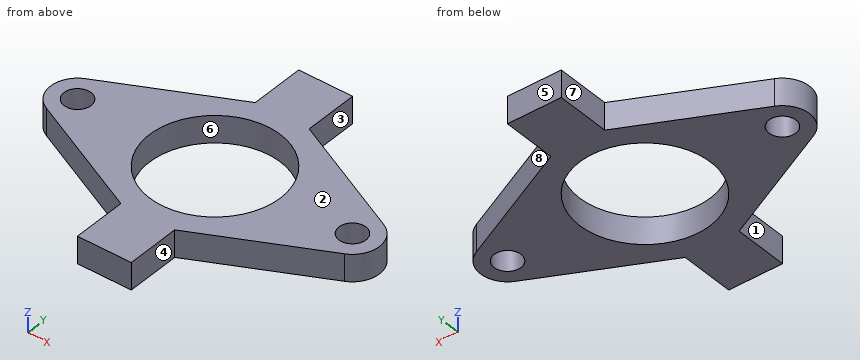
from build123d import *

# Parameters (mm, degrees)
SKETCH1_R           = 24.25
SKETCH1_R_2         = 5
BOSS_EXTRUDE1_DEPTH = 10


with BuildPart() as part:
    # Sketch1 → Boss-Extrude1 (new body)
    with BuildSketch(Plane.XY):
        with BuildLine():
            Line((10, 54.25), (-10, 54.25))
            Line((-10, 54.25), (-10, 34.25))
            Line((-10, 34.25), (-55.400247003, 12.302884399))
            ThreePointArc((-55.400247003, 12.302884399), (-61.047971586, 3.299679487), (-55.400247003, -5.703525425))
            Line((-55.400247003, -5.703525425), (-10, -27.650641026))
            Line((-10, -27.650641026), (-10, -47.650641026))
            Line((-10, -47.650641026), (10, -47.650641026))
            Line((10, -47.650641026), (10, -27.650641026))
            Line((10, -27.650641026), (55.400247003, -5.703525425))
            ThreePointArc((55.400247003, -5.703525425), (61.047971586, 3.299679487), (55.400247003, 12.302884399))
            Line((55.400247003, 12.302884399), (10, 34.25))
            Line((10, 34.25), (10, 54.25))
        make_face()
        with Locations((0, 3.299679487)):
            Circle(SKETCH1_R, mode=Mode.SUBTRACT)
        with Locations((51.047971586, 3.299679487)):
            Circle(SKETCH1_R_2, mode=Mode.SUBTRACT)
        with Locations((-51.047971586, 3.299679487)):
            Circle(SKETCH1_R_2, mode=Mode.SUBTRACT)
    extrude(amount=-BOSS_EXTRUDE1_DEPTH)


solid = part.part
Geometry: final body of the model. Coordinates: model frame, mm. Face numbers are marked on the shaded views. A direction names the side the tool comes from. Coordinates: 2 decimals unless noted, no trailing zeros. Write each loop counter-clockwise with the first axis right and the second up, starting at its lowest first coordinate (ties: lowest second). Pieces come first, ordered by that corner, then holes. Notation, with made-up numbers: (37, 48) - (70, 48) arc R5 ccw to (70, 55) - close; hole circle Ø3 at (-38, -32.5). An arc over 180 degrees is marked (long way). Return JSON: item names as keys, results as strings.
Item 1: Pull-direction query (X, two-part tool) for the marked faces 6, 7 and 8; classes: +X half, -X half, draft (parallel to the pull), parting line (faces both ways), or undercut.
Completed:
{"face 6": "undercut", "face 7": "-X half", "face 8": "+X half"}
Item 2: Pin query (flat end, axial travel): pin 1 Ø3 at (y, z) = (39.5, -7) entering from -X; pin 2 Ø2 at (y, z) = (-1, -6.5) entering from +X; pin 3 Ø1 at (x, z) = (33.5, -8.5) entering from -Y; pin 4 Ø6 at (x, y) = (51.05, 3.3) entering from -Z. Return the tip coordinate at first contact, or that it passes through.
Completed:
{"pin 1": "stops at x = -10", "pin 2": "stops at x = 60.49", "pin 3": "stops at y = -16.53", "pin 4": "passes through"}
Item 3: Line query: L1, parallel to X at y = 3, z = -2; L2, parallel to Y at x = 0, z = -2.5; L3, parallel to X at y = 47, z = -5.75. Output: solid intervals per line, ascending.
Completed:
{"L1": "x = -61.04 to -56.04, -46.06 to -24.25, 24.25 to 46.06, 56.04 to 61.04", "L2": "y = -47.65 to -20.95, 27.55 to 54.25", "L3": "x = -10 to 10"}
Item 4: Reachability of the marked faces 1, 2, 3, 4 and 5 from +Z, -Z, +X, -X, +Y, -Y: full face, straight path, thin tool, end or side. Return the list, or none.
Completed:
{"face 1": "+Z, -Z, -X, -Y", "face 2": "+Z, +X, -X, +Y, -Y", "face 3": "+Z, -Z, +X, +Y", "face 4": "+Z, -Z, +X, -Y", "face 5": "+Z, -Z, +X, -X, +Y"}
Item 5: Section query B-B (y = -13). Output: boundary loops of the cut face in (x, z).
Completed:
{"outline": "(-40.31, -10) - (-17.96, -10) - (-17.96, 0) - (-40.31, 0) - close; (17.96, -10) - (40.31, -10) - (40.31, 0) - (17.96, 0) - close"}
Item 6: Section query C-C (y = 6.5). Output: boundary loops of the cut face in (x, z).
Completed:
{"outline": "(-60.52, -10) - (-54.89, -10) - (-54.89, 0) - (-60.52, 0) - close; (-47.21, -10) - (-24.04, -10) - (-24.04, 0) - (-47.21, 0) - close; (24.04, -10) - (47.21, -10) - (47.21, 0) - (24.04, 0) - close; (54.89, -10) - (60.52, -10) - (60.52, 0) - (54.89, 0) - close"}
Item 7: Section query D-D (z = -8.25). Output: boundary loops of the cut face in (x, y), and give its area (3 significant figures).
Completed:
{"outline": "(-55.4, -5.7) - (-10, -27.65) - (-10, -47.65) - (10, -47.65) - (10, -27.65) - (55.4, -5.7) arc R10 ccw to (55.4, 12.3) - (10, 34.25) - (10, 54.25) - (-10, 54.25) - (-10, 34.25) - (-55.4, 12.3) arc R10 ccw to start; hole circle Ø10 at (-51.05, 3.3); hole circle Ø48.5 at (0, 3.3); hole circle Ø10 at (51.05, 3.3)", "area": "3,810 mm2"}
Item 8: Section query A-A (x = 0). Output: boundary loops of the cut face in (y, z), and give its area (3 significant figures).
Completed:
{"outline": "(-47.65, -10) - (-20.95, -10) - (-20.95, 0) - (-47.65, 0) - close; (27.55, -10) - (54.25, -10) - (54.25, 0) - (27.55, 0) - close", "area": "534 mm2"}
